Study the drawing (mm; zero at the part's minimum x, y, z) and answer. A direction names the side the tool comes from. Round coordinates to 2 decimals unless told otherwise and drop trailing zeros. Write each loop counter-clockwise with the first axis right and the second up, starting at its lowest first coordinate (ties: lowest second). Pieces come first, ordered by that corner, then holes. Notation, with made-up numbers: (-40, -18.75) -> (-24, -18.75) arc R25 cw to (-24, 13.25) -> close; hole circle Ø9 at (-15, 1.5). An arc over 180 degrees is marked (long way). Write each question's results on one line, items separated by ' | '. Start each with the question number.
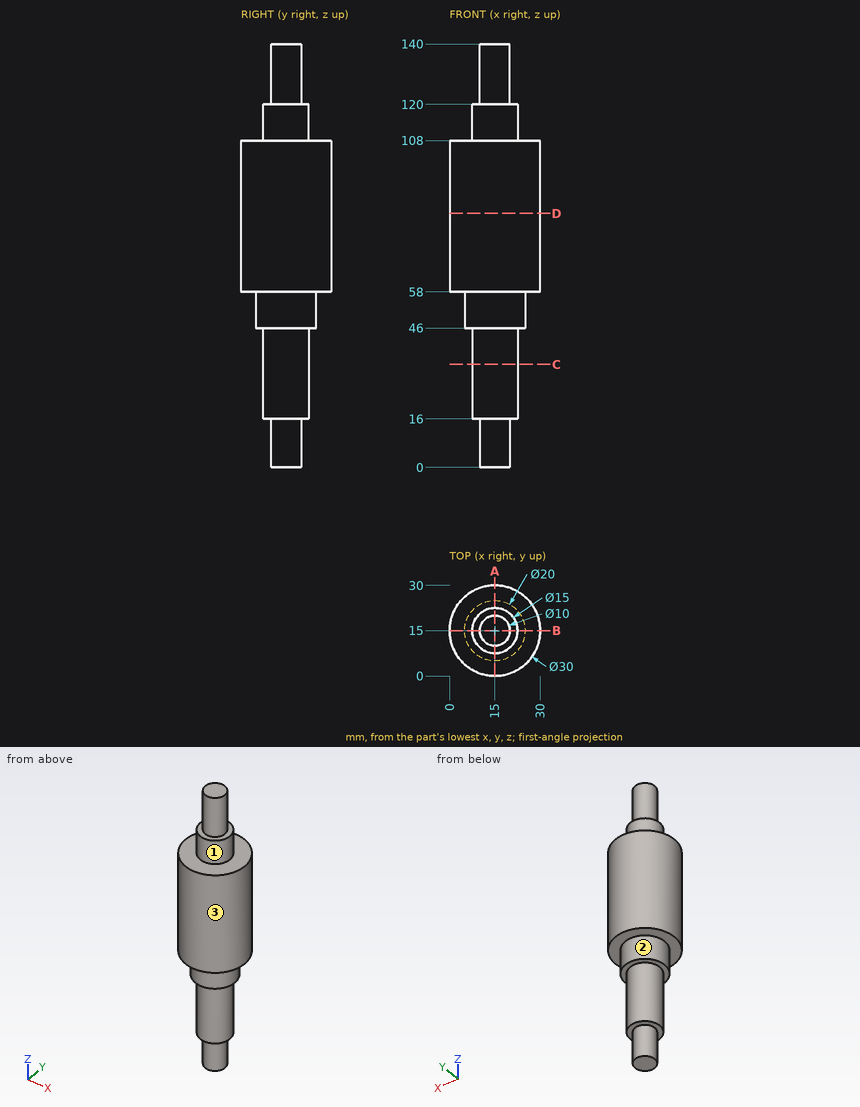
Q1. The part is cut by section D-D, the plane z = 84. Write down the section's boundary in (x, y), then the cut area to 3 significant figures.
Q2. The part is cut by section C-C, the plane z = 34. Write down the section's boundary in (x, y), then the cut area to 3 significant figures.
Q3. For the marked faces 1, 2 and 3, determine the directions among +Z, -Z, +X, -X, +Y, -Y from which every point of the face is accessible in a straight line to the end or side of a thin tool.
Q4. The part is cut by section A-A, the plane x = 15. Write down the section's boundary in (y, z).
Q5. Find the intervals of material crossed by line 1 (X direction, y = 2, z = 70); line 2 (Z direction, x = 15.5, y = 27.75); line 3 (Z direction, x = 21.5, y = 19.5), in increasing order.
Q6. Each of these flat-tipped pins is pushed along its axis until it touches: pin 1 (1 mm diameter, centred on x = 24.5, z = 51.5, fed in from -Y); pin 2 (3 mm diameter, centred on y = 18, z = 98, fed in from -X); pin 3 (8 mm diameter, centred on x = 3.5, y = 17, fed in from -Z); pin 4 (6 mm diameter, centred on x = 26, z = 35, fed in from -Y). Where does it stop, or does it pass through?
Answers follow:
1) outline: circle Ø30 at (15, 15) | area: 707 mm^2
2) outline: circle Ø15 at (15, 15) | area: 177 mm^2
3) face 1: +Z | face 2: -Z | face 3: +Z, -Z
4) outline: (0, 58) -> (5, 58) -> (5, 46) -> (7.5, 46) -> (7.5, 16) -> (10, 16) -> (10, 0) -> (20, 0) -> (20, 16) -> (22.5, 16) -> (22.5, 46) -> (25, 46) -> (25, 58) -> (30, 58) -> (30, 108) -> (22.5, 108) -> (22.5, 120) -> (20, 120) -> (20, 140) -> (10, 140) -> (10, 120) -> (7.5, 120) -> (7.5, 108) -> (0, 108) -> close
5) line 1: 7.52 to 22.48 | line 2: 58 to 108 | line 3: 46 to 108
6) pin 1: y = 10.64 | pin 2: x = 0.08 | pin 3: z = 46 | pin 4: through
